Input: part model. Units: mm. Frame: model coordinates. Give positions to 0.01 mm unless a question says otherwise; leave off trailing zeros. Write each loop counter-clockwise with the first axis right and the second up, starting at its lowest first coordinate (ties: lowest second). Pieces come first, ordered by that corner, then holes. Notation, with made-up numbers: (27.5, -14) -> (47.5, -14) arc R25 cw to (47.5, 25) -> close; hole circle Ø2 at (30.25, -28.5). An arc over 180 degrees is marked (long way). Answer as a JSON object with one key per item and string values. Group by question number.
from build123d import *

# Parameters (mm, degrees)
BOSS_EXTRUDE1_DEPTH = 0.75438


with BuildPart() as part:
    # Sketch1 → Boss-Extrude1 (new body)
    with BuildSketch(Plane.XY):
        with BuildLine():
            Line((-15, -35), (15, -35))
            Line((15, -35), (26.292884648, -14.44590658))
            ThreePointArc((26.292884648, -14.44590658), (0, 30), (-26.292884648, -14.44590658))
            Line((-26.292884648, -14.44590658), (-15, -35))
        make_face()
        with BuildLine():
            Line((-7.5, -23.848480035), (-7.5, -21.213203436))
            ThreePointArc((-7.5, -21.213203436), (0, 22.5), (7.5, -21.213203436))
            Line((7.5, -21.213203436), (7.5, -23.848480035))
            ThreePointArc((7.5, -23.848480035), (0, 25), (-7.5, -23.848480035))
        make_face(mode=Mode.SUBTRACT)
    extrude(amount=BOSS_EXTRUDE1_DEPTH)


solid = part.part
1. Section A-A (x = 0). Return the cut outline in (y, z), plus the area to 3 significant figures.
2. Section D-D (x = -11.5). Return the cut outline in (y, z), plus the area to 3 significant figures.
3. Section B-B (y = 0). Return the cut outline in (x, z).
4. Mould query, pull axis X, two halves, no side actions, for faces 1 (the face through (20.567, -24.867, 0.372)), 2 (the face through (0.99, 24.98, 0.37)), 3 (the face through (0, -2, 0.754)). Classes: pulls with the +X half, pulls with the -X half, needs draft (parallel to the pull), parting line crosses it, or undercut.
5. Line query: line 1 (X direction, y = 0, z = 0.2); line 2 (X direction, y = 3, z = 0.5); line 3 (Y direction, x = -12.5, z = 0.4). Output: solid intervals per line, ascending.
6. Section C-C (z = 0.25). Return the cut outline in (x, y).
Working result:
{
 "1": {"outline": "(-35, 0) -> (22.5, 0) -> (22.5, 0.75) -> (-35, 0.75) -> close; (25, 0) -> (30, 0) -> (30, 0.75) -> (25, 0.75) -> close", "area": "47.1 mm^2"},
 "2": {"outline": "(-35, 0) -> (-22.2, 0) -> (-22.2, 0.75) -> (-35, 0.75) -> close; (-19.34, 0) -> (19.34, 0) -> (19.34, 0.75) -> (-19.34, 0.75) -> close; (22.2, 0) -> (27.71, 0) -> (27.71, 0.75) -> (22.2, 0.75) -> close", "area": "43.0 mm^2"},
 "3": {"outline": "(-30, 0) -> (-25, 0) -> (-25, 0.75) -> (-30, 0.75) -> close; (-22.5, 0) -> (22.5, 0) -> (22.5, 0.75) -> (-22.5, 0.75) -> close; (25, 0) -> (30, 0) -> (30, 0.75) -> (25, 0.75) -> close"},
 "4": {"face 1": "pulls with the +X half", "face 2": "undercut", "face 3": "needs draft"},
 "5": {"line 1": "x = -30 to -25, -22.5 to 22.5, 25 to 30", "line 2": "x = -29.85 to -24.82, -22.3 to 22.3, 24.82 to 29.85", "line 3": "y = -35 to -21.65, -18.71 to 18.71, 21.65 to 27.27"},
 "6": {"outline": "(-26.29, -14.45) -> (-15, -35) -> (15, -35) -> (26.29, -14.45) arc R30 ccw (long way) to start; hole (-7.5, -23.85) -> (-7.5, -21.21) arc R22.5 cw (long way) to (7.5, -21.21) -> (7.5, -23.85) arc R25 ccw (long way) to start"}
}
